Model file for the job. Use its own axes, mm. Face numbers are marked on the shaded views. A direction names the side the tool comes from. Round coordinates to 2 decimals unless told otherwise and drop trailing zeros. Order: outer loops, then holes, each group sorted by start corner. A loop starts at its lowest first (then second) coordinate and runs counter-clockwise, first axis right, second up. Notation, with made-up numbers: (13.5, 44) - (63.5, 44) arc R22 cw to (63.5, 67) - close; hole circle Ø1 at (54.25, 83). An arc over 180 degrees is marked (long way). Use one line per item in the form item = value.
from build123d import *

# Parameters (mm, degrees)
SZKIC1_W                             = 40
SZKIC1_H                             = 40
DODANIE_WYCI_GNI_CIE1_DEPTH          = 5
OTWORY_USTALAJ_CE_3_0MM1_D           = 3
OTWORY_USTALAJ_CE_3_0MM1_CSINK_D     = 3.05
OTWORY_USTALAJ_CE_3_0MM1_CSINK_ANGLE = 90
SZKIC4_W                             = 32
SZKIC4_H                             = 6
DODANIE_WYCI_GNI_CIE2_DEPTH          = 40
OTWORY_USTALAJ_CE_3_0MM2_D           = 3
OTWORY_USTALAJ_CE_3_0MM2_CSINK_D     = 3.05
OTWORY_USTALAJ_CE_3_0MM2_CSINK_ANGLE = 90


with BuildPart() as part:
    # Szkic1 → Dodanie-wyciągnięcie1 (new body)
    with BuildSketch(Plane.XY):
        with Locations((20, 20)):
            Rectangle(SZKIC1_W, SZKIC1_H)
    extrude(amount=DODANIE_WYCI_GNI_CIE1_DEPTH)

    # Otwory ustalające Ø3.0mm1 (through all)
    with Locations(Plane.XY.offset(5)):
        with Locations((10.75, 29.25), (29.25, 29.25), (10.75, 10.75), (29.25, 10.75)):
            CounterSinkHole(OTWORY_USTALAJ_CE_3_0MM1_D / 2, OTWORY_USTALAJ_CE_3_0MM1_CSINK_D / 2, counter_sink_angle=OTWORY_USTALAJ_CE_3_0MM1_CSINK_ANGLE)

    # Szkic4 → Dodanie-wyciągnięcie2 (add)
    with BuildSketch(Plane.XY.offset(5)):
        with Locations((20, 3)):
            Rectangle(SZKIC4_W, SZKIC4_H)
    extrude(amount=DODANIE_WYCI_GNI_CIE2_DEPTH)

    # Otwory ustalające Ø3.0mm2 (through all)
    with Locations(Plane(origin=(0, 6, 0), x_dir=(1, 0, 0), z_dir=(0, 1, 0))):
        with Locations((7.5, -41.5), (32.5, -41.5)):
            CounterSinkHole(OTWORY_USTALAJ_CE_3_0MM2_D / 2, OTWORY_USTALAJ_CE_3_0MM2_CSINK_D / 2, counter_sink_angle=OTWORY_USTALAJ_CE_3_0MM2_CSINK_ANGLE)


solid = part.part
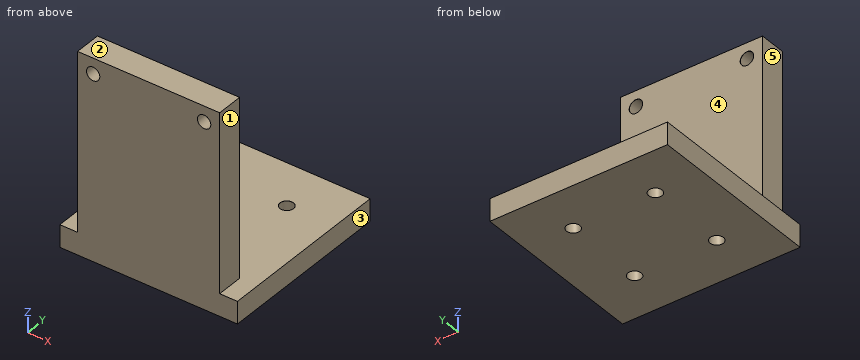
(1) Tool access for the marked faces 1, 2, 3, 4 and 5: list every direction of +Z, -Z, +X, -X, +Y, -Y with a clear straight run to the whole face (end or side of a thin tool).
Report:
face_1 = +Z, +X, +Y, -Y
face_2 = +Z, +X, -X, +Y, -Y
face_3 = +Z, -Z, +X, +Y, -Y
face_4 = +Z, +X, -X, +Y
face_5 = +Z, -X, +Y, -Y
(2) Slice it at D-D on z = 23.5. Give the cut face in (x, y).
Report:
outline = (4, 0) - (36, 0) - (36, 6) - (4, 6) - close
(3) Pin check, flat tips, straight feed: pin 1 (12 mm diameter, centred on x = 28.5, y = 18, fed in from +Z); pin 2 (2.5 mm diameter, centred on x = 10.75, y = 29.25, fed in from -Z); pin 3 (1.8 mm diameter, centred on y = 4, z = 34.5, fed in from -X); pin 4 (6.5 mm diameter, centred on y = 3, z = 29.5, fed in from +X). Stop position of each tip, or through.
Report:
pin_1 = 5
pin_2 = through
pin_3 = 4
pin_4 = 36
(4) Slice it at B-B on y = 29.25. Give the cut face in (x, z) (3 decimals), then the cut area to 3 significant figures.
Report:
outline = (0, 0) - (9.25, 0) - (9.25, 4.975) - (9.225, 5) - (0, 5) - close; (12.25, 0) - (27.75, 0) - (27.75, 4.975) - (27.725, 5) - (12.275, 5) - (12.25, 4.975) - close; (30.75, 0) - (40, 0) - (40, 5) - (30.775, 5) - (30.75, 4.975) - close
area = 170 mm2
(5) Slice it at A-A on x = 29.25. Give the cut face in (y, z) (3 decimals).
Report:
outline = (0, 0) - (9.25, 0) - (9.25, 4.975) - (9.225, 5) - (6, 5) - (6, 45) - (0, 45) - close; (12.25, 0) - (27.75, 0) - (27.75, 4.975) - (27.725, 5) - (12.275, 5) - (12.25, 4.975) - close; (30.75, 0) - (40, 0) - (40, 5) - (30.775, 5) - (30.75, 4.975) - close
(6) Slice it at C-C on z = 41.5. Give the cut face in (x, y) (3 decimals), then the cut area to 3 significant figures.
Report:
outline = (4, 0) - (6, 0) - (6, 5.975) - (5.975, 6) - (4, 6) - close; (9, 0) - (31, 0) - (31, 5.975) - (30.975, 6) - (9.025, 6) - (9, 5.975) - close; (34, 0) - (36, 0) - (36, 6) - (34.025, 6) - (34, 5.975) - close
area = 156 mm2
(7) Probe probe 1 along X at (y, z) = (3.25, 41.5); probe 2 along Y at (x, z) = (29.25, 2.15); probe 3 along Z at (x, y) = (32.5, 1.4). List the from-to ranges inside material, lowest first. Write a range as [from, to].
Report:
probe_1 = [4, 6], [9, 31], [34, 36]
probe_2 = [0, 9.25], [12.25, 27.75], [30.75, 40]
probe_3 = [0, 40], [43, 45]
